Model file for the job. Use its own axes, mm. Face numbers are marked on the shaded views. A direction names the side the tool comes from. Coordinates: 2 decimals unless noted, no trailing zeros. Order: outer loops, then holes, each group sorted by start corner. A loop starts at its lowest first (then second) coordinate and runs counter-clockwise, first axis right, second up. Notation, with made-up numbers: M 29.25,-27.75 L 78.25,-27.75 A20 cw 78.25,-17.75 Z; hole C 48,-32 d9. An arc over 180 degrees is marked long. Return JSON: item names as keys, results as strings.
```python
from build123d import *

# Parameters (mm, degrees)
DISQUE_INT_RIEUR_W              = 2
DISQUE_INT_RIEUR_H              = 9
DISQUE_EXT_RIEUR_W              = 2
DISQUE_EXT_RIEUR_H              = 9
DISQUE_INTERM_DIAIRE_W          = 4.5
DISQUE_INTERM_DIAIRE_H          = 7
CONG_1_DISQUE_EXT_RIEUR_0_5MM_R = 0.5


with BuildPart() as part:
    # Disque_Int_rieur → R_volution1_Disque_Int_rieur (revolve)
    with BuildSketch(Plane.XY, mode=Mode.PRIVATE) as r_volution1_disque_int_rieur_sk:
        with Locations((8.5, 0)):
            Rectangle(DISQUE_INT_RIEUR_W, DISQUE_INT_RIEUR_H)
    revolve(r_volution1_disque_int_rieur_sk.sketch.rotate(Axis((0, 4.95, 0), (0, -1, 0)), 90), axis=Axis((0, 4.95, 0), (0, -1, 0)))



with BuildPart() as body_2:
    # Disque_ext_rieur → R_volution2_Disque_ext_rieur (revolve)
    with BuildSketch(Plane.XY, mode=Mode.PRIVATE) as r_volution2_disque_ext_rieur_sk:
        with Locations((15, 0)):
            Rectangle(DISQUE_EXT_RIEUR_W, DISQUE_EXT_RIEUR_H)
    revolve(r_volution2_disque_ext_rieur_sk.sketch.rotate(Axis((0, 4.95, 0), (0, -1, 0)), 90), axis=Axis((0, 4.95, 0), (0, -1, 0)))


with BuildPart() as part_1:
    add(part.part)

    add(body_2.part)  # R_volution3_Disque_Interm_diaire merges body 2
    # Disque_Interm_diaire → R_volution3_Disque_Interm_diaire (revolve)
    with BuildSketch(Plane.XY, mode=Mode.PRIVATE) as r_volution3_disque_interm_diaire_sk:
        with Locations((11.75, 0)):
            Rectangle(DISQUE_INTERM_DIAIRE_W, DISQUE_INTERM_DIAIRE_H)
    revolve(r_volution3_disque_interm_diaire_sk.sketch.rotate(Axis((0, 4.95, 0), (0, -1, 0)), 90), axis=Axis((0, 4.95, 0), (0, -1, 0)))

    # Cong_1_Disque_ext_rieur_0.5mm
    cong_1_disque_ext_rieur_0_5mm_edges = [part_1.edges().sort_by_distance(p)[0] for p in [
        (0, -4.5, -16),
        (0, 4.5, -16),
    ]]
    fillet(cong_1_disque_ext_rieur_0_5mm_edges, radius=CONG_1_DISQUE_EXT_RIEUR_0_5MM_R)


solid = part_1.part
```
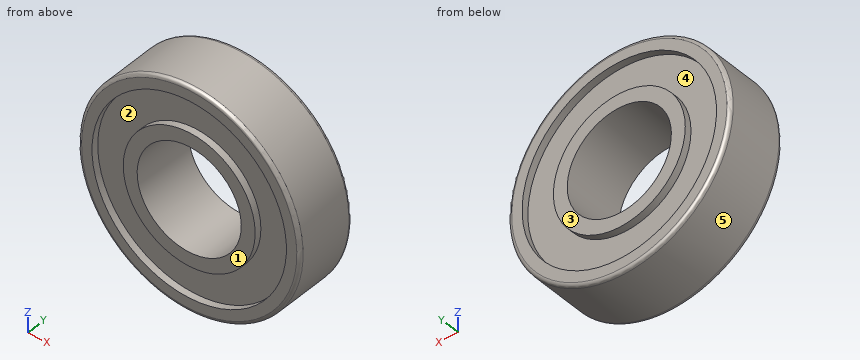
Item 1: 3-axis set-ups, long thin cutter, end or side, ignore diameter. For the marked faces 1 and 2: which of +Z, -Z, +X, -X, +Y, -Y reach the whole face in a straight line?
Check result:
{"face 1": "+Z, -Z, +X, -X, -Y", "face 2": "-Y"}
Item 2: Pull direction X, two halves, no side cores. Call the marked faces 3, 4 and 5: +X half, -X half, draft (parallel to the pull), parting line (faces both ways), or undercut.
Check result:
{"face 3": "draft", "face 4": "undercut", "face 5": "parting line"}
Item 3: Saw through at C-C (y = -0.5). Write the cut outline in (x, z).
Check result:
{"outline": "C 0,0 d32; hole C 0,0 d15"}
Item 4: Saw through at A-A (z = 0). Write the cut outline in (x, y), and give its area (3 significant figures).
Check result:
{"outline": "M -16,-4 A0.5 ccw -15.5,-4.5 L -14,-4.5 L -14,-3.5 L -9.5,-3.5 L -9.5,-4.5 L -7.5,-4.5 L -7.5,4.5 L -9.5,4.5 L -9.5,3.5 L -14,3.5 L -14,4.5 L -15.5,4.5 A0.5 ccw -16,4 Z; M 7.5,-4.5 L 9.5,-4.5 L 9.5,-3.5 L 14,-3.5 L 14,-4.5 L 15.5,-4.5 A0.5 ccw 16,-4 L 16,4 A0.5 ccw 15.5,4.5 L 14,4.5 L 14,3.5 L 9.5,3.5 L 9.5,4.5 L 7.5,4.5 Z", "area": "135 mm2"}
Item 5: Drop flat-ended pins along their axis: pin 1 Ø2 at (x, y) = (11.5, 0) entering from -Z; pin 2 Ø13.5 at (x, z) = (0, 0) entering from -Y. Give the stop position or say it passes through.
Check result:
{"pin 1": "stops at z = -12.07", "pin 2": "passes through"}
Item 6: Saw through at B-B (x = 0). Write the cut outline in (y, z), and give its area (3 significant figures).
Check result:
{"outline": "M -4.5,-15.5 A0.5 ccw -4,-16 L 4,-16 A0.5 ccw 4.5,-15.5 L 4.5,-14 L 3.5,-14 L 3.5,-9.5 L 4.5,-9.5 L 4.5,-7.5 L -4.5,-7.5 L -4.5,-9.5 L -3.5,-9.5 L -3.5,-14 L -4.5,-14 Z; M -4.5,7.5 L 4.5,7.5 L 4.5,9.5 L 3.5,9.5 L 3.5,14 L 4.5,14 L 4.5,15.5 A0.5 ccw 4,16 L -4,16 A0.5 ccw -4.5,15.5 L -4.5,14 L -3.5,14 L -3.5,9.5 L -4.5,9.5 Z", "area": "135 mm2"}
Item 7: Wall check: line 1 (X direction, y = -4.05, z = 0); line 2 (Z direction, x = -5.5, y = -1.75); line 3 (X direction, y = -2.75, z = -6.5). Give the ranges that are in metal, low to high.
Check result:
{"line 1": "x = -16 to -14, -9.5 to -7.5, 7.5 to 9.5, 14 to 16", "line 2": "z = -15.02 to -5.1, 5.1 to 15.02", "line 3": "x = -14.62 to -3.74, 3.74 to 14.62"}
